from build123d import *

# Parameters (mm, degrees)
F0_W     = 558.8
F0_H     = 558.8
F1_DEPTH = 12.7
F2_W     = 368.3
F2_H     = 368.3
F3_DEPTH = 20.32
F4_W     = 336.55
F4_H     = 336.55
F5_DEPTH = 121.92


with BuildPart() as f1:
    # F0 (on Top) → F1 (new body)
    with BuildSketch(Plane.XY):
        Rectangle(F0_W, F0_H)
    extrude(amount=F1_DEPTH)

    # F2 (on face) → F3 (join)
    with BuildSketch(Plane.XY.offset(12.7)):
        Rectangle(F2_W, F2_H)
    extrude(amount=F3_DEPTH)

    # F4 (on face) → F5 (cut)
    with BuildSketch(Plane.XY.offset(33.02)):
        Rectangle(F4_W, F4_H)
    extrude(amount=-F5_DEPTH, mode=Mode.SUBTRACT)


solid = f1.part
The model under review builds one solid part; all positions refer to its coordinate system, in mm. A direction names the side the tool comes from. Round coordinates to 2 decimals unless told otherwise and drop trailing zeros. Loops run counter-clockwise (first coordinate to the right, second up) from the corner with the lowest first, then second, coordinate; pieces in that order, holes last. Notation, with made-up numbers: M 35,1.25 L 77,1.25 A13 cw 77,10.25 Z; hole C 76.5,6 d1. An arc over 180 degrees is marked long. Answer as a JSON object with one key per item and string values.
Item 1: We need section D-D, the plane x = -193. State the section outline as (y, z) points, and give its area (3 significant figures).
Check sheet entries:
{"outline": "M -279.4,0 L 279.4,0 L 279.4,12.7 L -279.4,12.7 Z", "area": "7,100 mm2"}
Item 2: The part is to be moulded in two halves that separate along Y. For faces 1 (the face through (-190, 4, 12.7)), 2 (the face through (-4, 279.4, 6)), 3 (the face through (-2, -168.275, 17)), say which applies: +Y half, -Y half, draft (parallel to the pull), parting line (faces both ways), or undercut.
Check sheet entries:
{"face 1": "draft", "face 2": "+Y half", "face 3": "undercut"}
Item 3: We need section A-A, the plane x = 91. State the section outline as (y, z) points (3 decimals), and give its area (3 significant figures).
Check sheet entries:
{"outline": "M -279.4,0 L -168.275,0 L -168.275,33.02 L -184.15,33.02 L -184.15,12.7 L -279.4,12.7 Z; M 168.275,0 L 279.4,0 L 279.4,12.7 L 184.15,12.7 L 184.15,33.02 L 168.275,33.02 Z", "area": "3,470 mm2"}
Item 4: Clearance check with flat-ended pins moving along their axes: P1, Ø2, axis at x = -139.5, z = 17, coming from the +Y side; P2, Ø6, axis at y = 3.5, z = 25, coming from the +X side; P3, Ø6, axis at y = 75, z = 24, coming from the -X side. State where each tip first meets the part, or that it passes through.
Check sheet entries:
{"P1": "y = 184.15", "P2": "x = 184.15", "P3": "x = -184.15"}
Item 5: For line 1 along Y through (x, z) = (-9, 22) (3 decimals); line 2 along X through (y, z) = (-120, 5) (3 decimals), list the stretches that pass through material, from the lowest coordinate up.
Check sheet entries:
{"line 1": "-184.15 to -168.275, 168.275 to 184.15", "line 2": "-279.4 to -168.275, 168.275 to 279.4"}
Item 6: Tool access review of faces 4 (the face through (-184.15, -3, 23)), 5 (the face through (168.275, -2, 17)), 6 (the face through (-3, -184.15, 23)), 7 (the face through (184.15, -3, 23)), 8 (the face through (-3, 184.15, 23)): name each direction out of +Z, -Z, +X, -X, +Y, -Y from which nothing blocks a thin tool from reaching the whole face with its end or side.
Check sheet entries:
{"face 4": "+Z, -X, +Y, -Y", "face 5": "+Z, -Z", "face 6": "+Z, +X, -X, -Y", "face 7": "+Z, +X, +Y, -Y", "face 8": "+Z, +X, -X, +Y"}
Item 7: We need section C-C, the plane z = 26. State the section outline as (x, y) points (3 decimals).
Check sheet entries:
{"outline": "M -184.15,-184.15 L 184.15,-184.15 L 184.15,184.15 L -184.15,184.15 Z; hole M -168.275,-168.275 L 168.275,-168.275 L 168.275,168.275 L -168.275,168.275 Z"}
